Can you work these out from the drawing? Everything is in mm from the part's minimum corner. A direction names the side the tool comes from. Round coordinates to 2 decimals unless told otherwise and drop trailing zeros. Write each loop counter-clockwise with the first axis right and the second up, starting at its lowest first coordinate (ties: lowest second). Pieces come first, ordered by that corner, then holes. Notation, with made-up numbers: (-2.75, 56.25) - (20.25, 56.25) arc R24 cw to (20.25, 66.25) - close; hole circle Ø10 at (15, 23.25). An arc over 180 degrees is marked (long way). Write each question's results on one line, items separated by ' | '. Start each with the question number.
(1) Imagine slicing it at C-C on y = 17. Write out the boundary of the cut face in (x, z), then the cut area to 3 significant figures.
(2) Imagine slicing it at B-B on z = 5. Write out the boundary of the cut face in (x, y).
(3) Imagine slicing it at D-D on x = 6.5. Write out the boundary of the cut face in (y, z), then the cut area to 3 significant figures.
(4) Thinking about a two-plate mould opening in Z: for the marked faces 1, 2 and 3, which applies, +Z half, -Z half, draft (parallel to the pull), parting line (faces both ways), or undercut?
(5) For P1, Ø6, axis at x = 2, z = 15, coming from the +Y side; P2, Ø8, axis at x = 10, y = 17, coming from the +Z side; P3, Ø12, axis at y = 15.5, z = 17.5, coming from the +X side, each with a flat end and sliding along its axis, tell me the tip position at first contact or that it passes through.
(6) On a 3-axis mill with a long thin cutter (end or side, diameter ignored), from which of +Z, -Z, +X, -X, +Y, -Y can I reach the whole of each face in a straight line? I mean the marked faces 4 and 5. Say none if no direction works.
(7) Please list where these lines run through material, in increasing order: line 1 (Y direction, x = 10, z = 2.5); line 2 (Y direction, x = 18, z = 12). Write a range as [from, to].
(8) Imagine slicing it at A-A on x = 10. Write out the boundary of the cut face in (y, z), then the cut area to 3 significant figures.
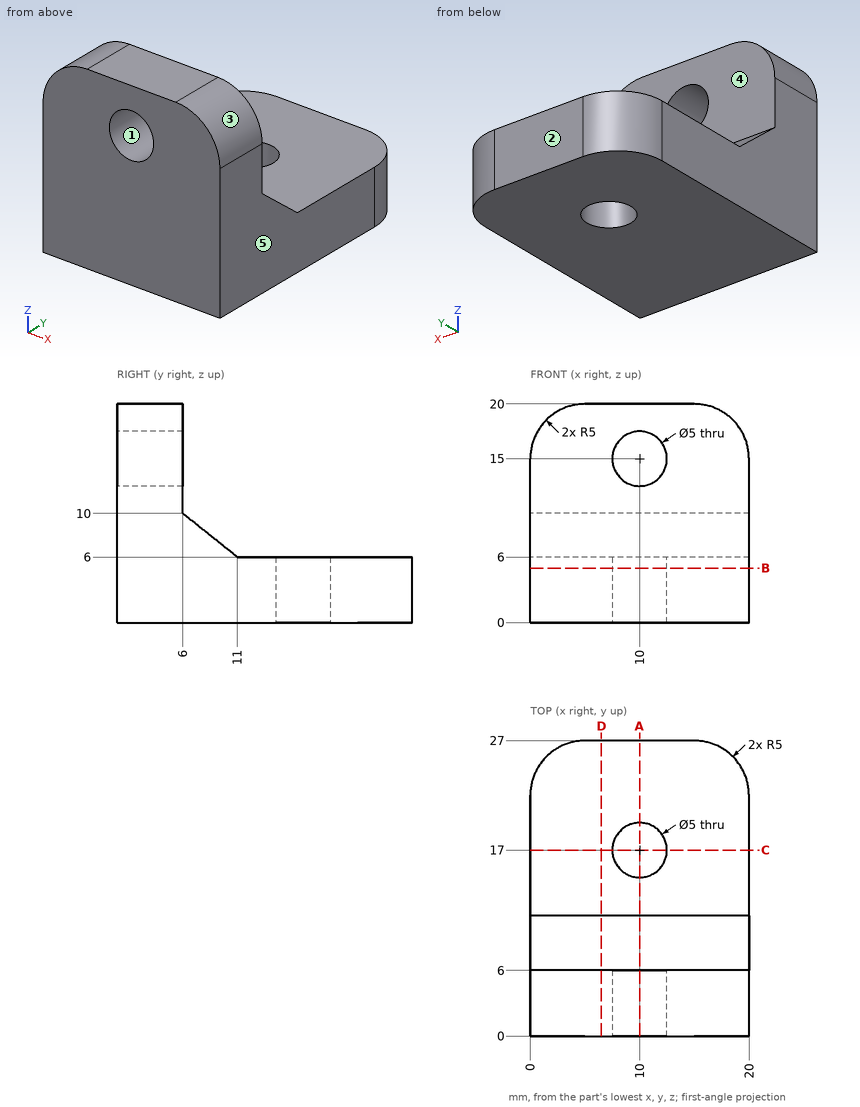
Response:
1) outline: (0, 0) - (7.5, 0) - (7.5, 6) - (0, 6) - close; (12.5, 0) - (20, 0) - (20, 6) - (12.5, 6) - close | area: 90.0 mm²
2) outline: (0, 0) - (20, 0) - (20, 22) arc R5 ccw to (15, 27) - (5, 27) arc R5 ccw to (0, 22) - close; hole circle Ø5 at (10, 17)
3) outline: (0, 0) - (27, 0) - (27, 6) - (11, 6) - (6, 10) - (6, 20) - (0, 20) - close | area: 256 mm²
4) face 1: undercut | face 2: draft | face 3: +Z half
5) P1: y = 6 | P2: z = 6 | P3: through
6) face 4: +Z, +X, -X, +Y | face 5: +Z, -Z, +X, +Y, -Y
7) line 1: [0, 14.5], [19.5, 27] | line 2: [0, 6]
8) outline: (0, 0) - (14.5, 0) - (14.5, 6) - (11, 6) - (6, 10) - (6, 12.5) - (0, 12.5) - close; (0, 17.5) - (6, 17.5) - (6, 20) - (0, 20) - close; (19.5, 0) - (27, 0) - (27, 6) - (19.5, 6) - close | area: 196 mm²
